Study the drawing (mm; zero at the part's minimum x, y, z) and answer. A direction names the side the tool comes from. Give positions to 0.01 mm unless a question says otherwise; leave off trailing zeros. Write each loop counter-clockwise with the first axis right and the second up, starting at its lowest first coordinate (ties: lowest second). Pieces come first, ordered by that corner, then holes. Notation, with made-up numbers: (-14.75, 35) - (20.25, 35) arc R22 cw to (20.25, 68) - close; hole circle Ø9 at (48, 78.5). An arc over 180 degrees is marked (long way). Write each question's results on one line, items separated by ' | '. Start each with the question number.
Q1. For the marked faces 4, 5 and 6, determine the directions among +Z, -Z, +X, -X, +Y, -Y from which every point of the face is accessible in a straight line to the end or side of a thin tool.
Q2. Flat-ended cylindrical pins translate along their axes: pin 1 Ø1 at (y, z) = (16, 1) entering from +X; pin 2 Ø4 at (x, z) = (13, 4.5) entering from -Y; pin 3 Ø1.5 at (x, z) = (3.5, 2.5) entering from -Y. Find the tip coordinate at first contact, or state that the pin passes through.
Q3. For a pull along Y with two mould halves and no side action, classify the marked faces 1, 2 and 3 as pulls with the +Y half, pulls with the -Y half, needs draft (parallel to the pull), parting line crosses it, or undercut.
Q4. Section C-C (z = 9) is taken. Determine the outline of the cut face in (x, y) (1 decimal).
Q5. Find the intervals of material crossed by probe 1 along Y at (x, z) = (16.51, 3.25); probe 2 along Z at (x, y) = (9.5, 30) (1 decimal); probe 3 along Y at (x, z) = (16, 1.25), in increasing order.
Q6. Section A-A (x = 16.51) is taken. Determine the outline of the cut face in (y, z) (1 decimal).
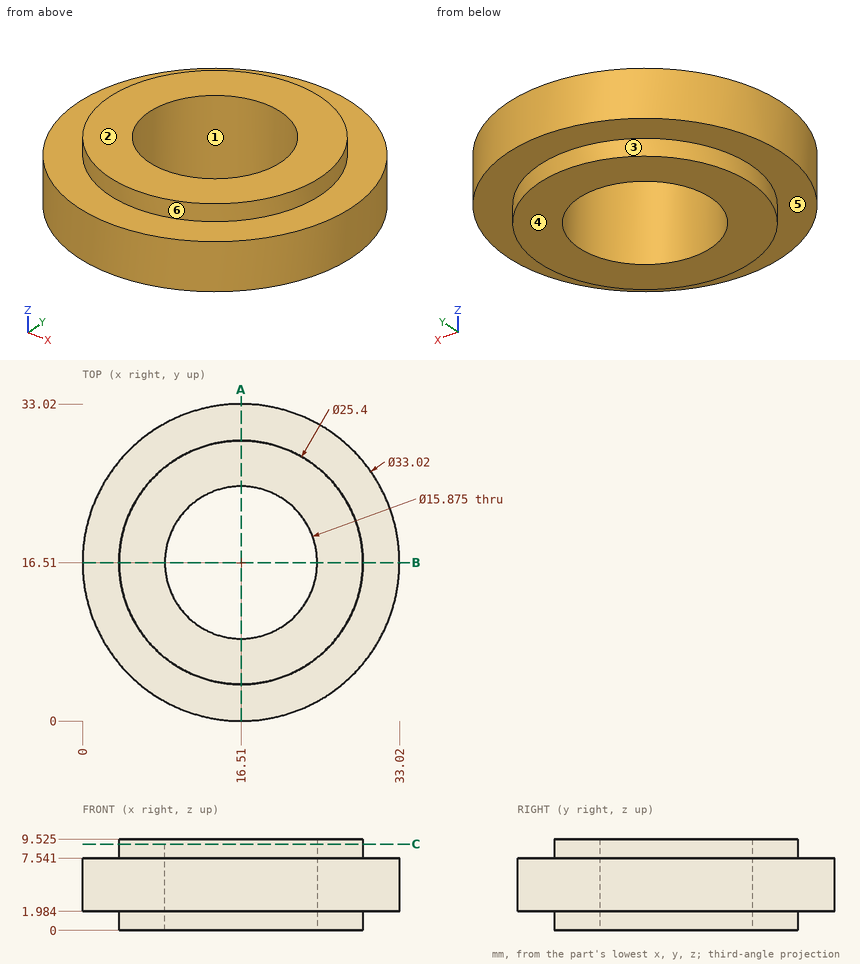
Answers below:
1) face 4: -Z, +X, -X, +Y, -Y | face 5: -Z | face 6: +Z
2) pin 1: stops at x = 29.21 | pin 2: stops at y = 0.07 | pin 3: stops at y = 5.45
3) face 1: undercut | face 2: needs draft | face 3: parting line crosses it
4) outline: circle Ø25.4 at (16.5, 16.5); hole circle Ø15.9 at (16.5, 16.5)
5) probe 1: y = 0 to 8.57, 24.45 to 33.02 | probe 2: z = 2 to 7.5 | probe 3: y = 3.82 to 8.59, 24.43 to 29.2
6) outline: (0, 2) - (3.8, 2) - (3.8, 0) - (8.6, 0) - (8.6, 9.5) - (3.8, 9.5) - (3.8, 7.5) - (0, 7.5) - close; (24.4, 0) - (29.2, 0) - (29.2, 2) - (33, 2) - (33, 7.5) - (29.2, 7.5) - (29.2, 9.5) - (24.4, 9.5) - close
